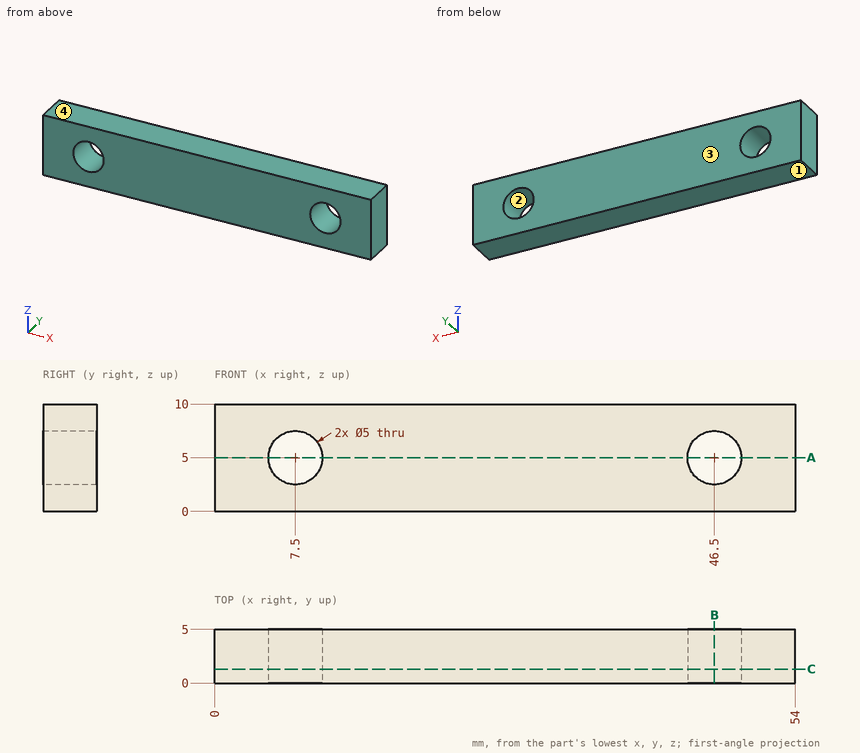
Could you check a few things on this drawing? It's one solid part, dimensions in mm from its lowest x, y, z. Coordinates: 2 decimals unless noted, no trailing zeros. Order: outer loops, then holes, each group sorted by start corner. A loop starts at its lowest first (then second) coordinate and runs counter-clockwise, first axis right, second up.
1. I need wall thicknesses on line 1 (X direction, y = 1.75, z = 5); line 2 (X direction, y = 1.65, z = 2.75); line 3 (Z direction, x = 47, y = 1.5). Which ranges of each line are inside material? Lowest first, please.
2. If we section it at B-B (x = 46.5): Please give me the cut outline in (y, z).
3. Thinking about a two-plate mould opening in Z: for the marked faces 1, 2, 3 and 4, which applies, +Z half, -Z half, draft (parallel to the pull), parting line (faces both ways), or undercut?
4. If we section it at A-A (z = 5): Please give me the cut outline in (x, y).
5. I'm going to push flat-ended pins straight in: pin 1 (3 mm diameter, centred on x = 19, z = 3, fed in from -Y); pin 2 (3 mm diameter, centred on x = 7.5, z = 5, fed in from -Y). Where does each tip first touch, or does it pass through?
6. If we section it at C-C (y = 1.3): Please give me the cut outline in (x, z).
Entries:
1. line 1: x = 0 to 5, 10 to 44, 49 to 54
1. line 2: x = 0 to 6.41, 8.59 to 45.41, 47.59 to 54
1. line 3: z = 0 to 2.55, 7.45 to 10
2. outline: (0, 0) - (5, 0) - (5, 2.5) - (0, 2.5) - close; (0, 7.5) - (5, 7.5) - (5, 10) - (0, 10) - close
3. face 1: -Z half
3. face 2: undercut
3. face 3: draft
3. face 4: +Z half
4. outline: (0, 0) - (5, 0) - (5, 5) - (0, 5) - close; (10, 0) - (44, 0) - (44, 5) - (10, 5) - close; (49, 0) - (54, 0) - (54, 5) - (49, 5) - close
5. pin 1: stops at y = 0
5. pin 2: passes through
6. outline: (0, 0) - (54, 0) - (54, 10) - (0, 10) - close; hole circle Ø5 at (7.5, 5); hole circle Ø5 at (46.5, 5)
